from build123d import *

# Parameters (mm, degrees)
BOSS_EXTRUDE2_DEPTH   = 8
M4_TAPPED_HOLE1_D     = 3.3
M4_TAPPED_HOLE1_DEPTH = 11.5
M4_TAPPED_HOLE1_TIP   = 0.991420021
SKETCH8_R             = 1.7
CUT_EXTRUDE1_DEPTH    = 10


with BuildPart() as part:
    # Sketch1 → Boss-Extrude2 (new body)
    with BuildSketch(Plane(origin=(0, 0, 0), x_dir=(1, 0, 0), z_dir=(0, 1, 0))):
        Polygon((35.397046685, 0.212206196), (35.397046685, -3.787793804), (-2.283249607, -3.787793804), (-2.283249607, -8.787793804), (-9.783249607, -8.787793804), (-18.892613672, -6.346947059), (-28.102933344, -8.814844777), (-34.602933344, -8.814844777), (-34.602933344, -4.117707659), (-27.103302555, 0.212206196), align=None)
    extrude(amount=BOSS_EXTRUDE2_DEPTH)

    # M4 Tapped Hole1
    with Locations(Plane(origin=(0, 0, -0.212206196), x_dir=(-1, 0, 0), z_dir=(0, 0, -1))):
        with Locations((18.892933344, 4)):
            Hole(M4_TAPPED_HOLE1_D / 2, depth=M4_TAPPED_HOLE1_DEPTH)
            with Locations((0, 0, -(M4_TAPPED_HOLE1_DEPTH + M4_TAPPED_HOLE1_TIP / 2))):  # 118° drill point
                Cone(0, M4_TAPPED_HOLE1_D / 2, M4_TAPPED_HOLE1_TIP, mode=Mode.SUBTRACT)

    # Sketch8 → Cut-Extrude1 (cut)
    with BuildSketch(Plane(origin=(0, 0, -0.212206196), x_dir=(-1, 0, 0), z_dir=(0, 0, -1))):
        with Locations((-31.397046685, 4)):
            Circle(SKETCH8_R)
        with Locations((-24.397046685, 4)):
            Circle(SKETCH8_R)
    extrude(amount=-CUT_EXTRUDE1_DEPTH, mode=Mode.SUBTRACT)


solid = part.part
Read the model definition and answer for the solid it produces. Units are mm, in the model's axes. A direction names the side the tool comes from. Give positions to 0.01 mm unless a question says otherwise; leave off trailing zeros. Write each loop counter-clockwise with the first axis right and the second up, starting at its lowest first coordinate (ties: lowest second). Pieces come first, ordered by that corner, then holes. Notation, with made-up numbers: (26, 23.5) -> (47, 23.5) arc R33 cw to (47, 54.5) -> close; hole circle Ø8 at (-17.75, -6.75). An arc over 180 degrees is marked (long way). Answer as a JSON object with one key per item and string values. Group by question number.
1) Find section C-C (x = 5). Write down the section's boundary in (y, z).
2) A tool of negligible diameter and unlimited length cuts with its end or side. For faces 1 (the flat face through (17, 4, 3.788)), 2 (the flat face through (-14.274, 3.944, 7.584)), 3 (the flat face through (-7, 8, 3)), from which of +Z, -Z, +X, -X, +Y, -Y can it reach the whole face along a straight path? Write none if from no direction.
3) Each of these flat-tipped pins is pushed along its axis until it touches: P1, Ø2.5, axis at x = 19, y = 4, coming from the +Z side; P2, Ø2.5, axis at y = 5, z = 5.5, coming from the +X side. Where does it stop, or does it pass through?
4) Consider L1, parallel to X at y = 3, z = 1.25; L2, parallel to Z at x = 19, y = 3.25; L3, parallel to Y at x = 24.5, z = 3.5. Determine where each line is inside the solid, lowest interval first. Write a range as from..to.
5) The mould has two halves that part along X. Classify faces 4 (the flat face through (4, 4, -0.212)), 5 (the flat face through (-2.283, 4, 6)), 6 (the flat face through (-23.433, 3.944, 7.564)): +X half, -X half, draft (parallel to the pull), parting line (faces both ways), or undercut.
6) Find section A-A (y = 5). Write down the section's boundary in (x, z), and give its area (3 significant figures).
7) Find section D-D (x = -16). Write down the section's boundary in (y, z), and give its area (3 significant figures).
8) Find section B-B (z = 2). Write down the section's boundary in (x, y).
Values follow:
{
 "1": {"outline": "(0, -0.21) -> (8, -0.21) -> (8, 3.79) -> (0, 3.79) -> close"},
 "2": {"face 1": "+Z, +X, +Y, -Y", "face 2": "+Z, +Y, -Y", "face 3": "+Z, -Z, +X, -X, +Y"},
 "3": {"P1": "stops at z = 3.79", "P2": "stops at x = -2.28"},
 "4": {"L1": "x = -29.64..-20.21, -17.58..23.02, 25.77..30.02, 32.77..35.4", "L2": "z = -0.21..3.79", "L3": "y = 0..2.3, 5.7..8"},
 "5": {"face 4": "draft", "face 5": "+X half", "face 6": "undercut"},
 "6": {"outline": "(-34.6, 4.12) -> (-27.1, -0.21) -> (-20.21, -0.21) -> (-20.21, 6.7) -> (-28.1, 8.81) -> (-34.6, 8.81) -> close; (-17.58, -0.21) -> (23.02, -0.21) -> (23.02, 3.79) -> (-2.28, 3.79) -> (-2.28, 8.79) -> (-9.78, 8.79) -> (-17.58, 6.7) -> close; (25.77, -0.21) -> (30.02, -0.21) -> (30.02, 3.79) -> (25.77, 3.79) -> close; (32.77, -0.21) -> (35.4, -0.21) -> (35.4, 3.79) -> (32.77, 3.79) -> close", "area": "364 mm2"},
 "7": {"outline": "(0, -0.21) -> (8, -0.21) -> (8, 7.12) -> (0, 7.12) -> close", "area": "58.7 mm2"},
 "8": {"outline": "(-30.93, 0) -> (35.4, 0) -> (35.4, 8) -> (-30.93, 8) -> close; hole circle Ø3.3 at (-18.89, 4); hole circle Ø3.4 at (24.4, 4); hole circle Ø3.4 at (31.4, 4)"}
}
